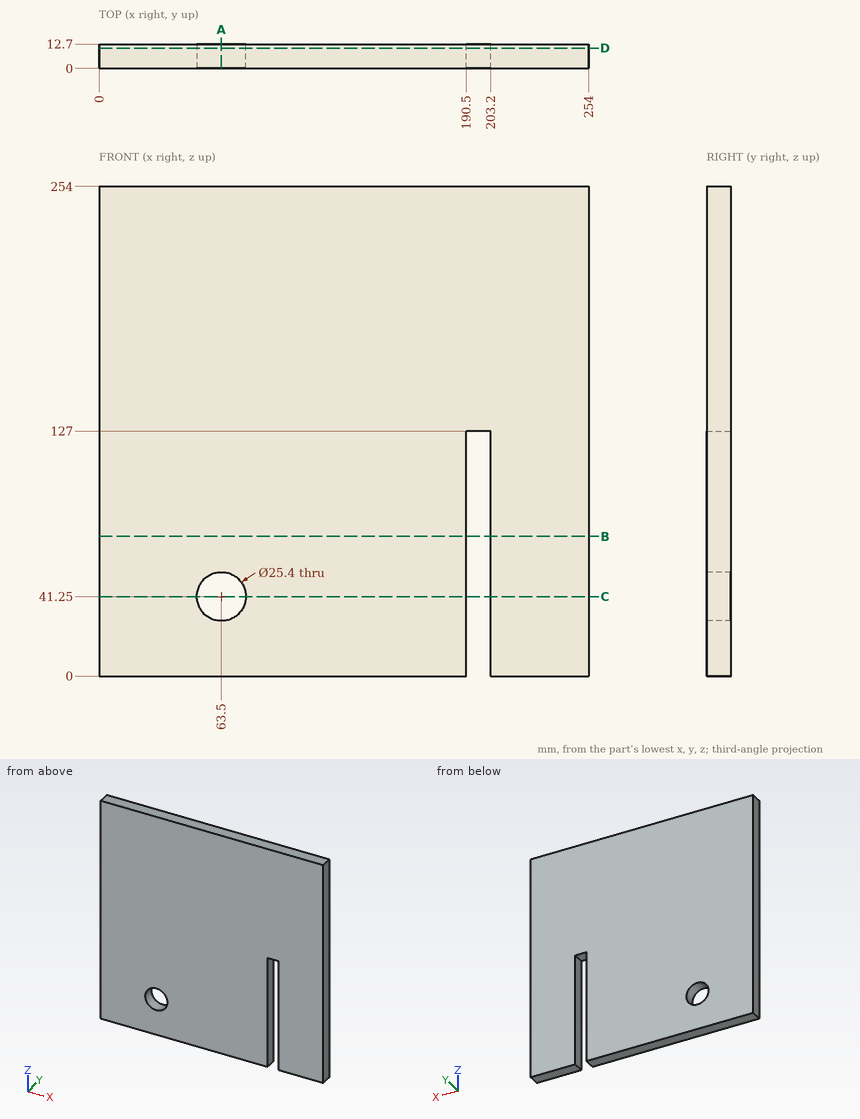
The figure shows three views and two pictorial views of one solid part (mm, origin at its lowest corner). Answer the questions. Coordinates: 2 decimals unless noted, no trailing zeros. Write each loop counter-clockwise with the first axis right and the second up, starting at its lowest first coordinate (ties: lowest second). Pieces come first, ordered by that corner, then holes. Notation, with made-up numbers: (-4, 61) -> (43, 61) arc R24 cw to (43, 71) -> close; hole circle Ø9 at (-38.75, 3). An arc over 180 degrees is marked (long way). Answer as a JSON object with one key per item and string values.
Q1. The part is cut by section A-A on x = 63.5. Give the vertices of the cut face in (y, z).
The answers:
{"outline": "(0, 0) -> (12.7, 0) -> (12.7, 28.55) -> (0, 28.55) -> close; (0, 53.95) -> (12.7, 53.95) -> (12.7, 254) -> (0, 254) -> close"}
Q2. Flat-ended cylindrical pins translate along their axes: pin 1 Ø20.5 at (x, z) = (63.5, 41.25) entering from -Y; pin 2 Ø6.5 at (x, y) = (199.5, 7) entering from -Z. Find the tip coordinate at first contact, or state that the pin passes through.
The answers:
{"pin 1": "passes through", "pin 2": "stops at z = 127"}
Q3. The part is cut by section B-B on z = 72.5. Give the vertices of the cut face in (x, y), then the cut area to 3 significant figures.
The answers:
{"outline": "(0, 0) -> (190.5, 0) -> (190.5, 12.7) -> (0, 12.7) -> close; (203.2, 0) -> (254, 0) -> (254, 12.7) -> (203.2, 12.7) -> close", "area": "3,060 mm2"}
Q4. The part is cut by section D-D on y = 10.5. Give the vertices of the cut face in (x, z), then the cut area to 3 significant figures.
The answers:
{"outline": "(0, 0) -> (190.5, 0) -> (190.5, 127) -> (203.2, 127) -> (203.2, 0) -> (254, 0) -> (254, 254) -> (0, 254) -> close; hole circle Ø25.4 at (63.5, 41.25)", "area": "62,400 mm2"}
Q5. The part is cut by section C-C on z = 41.25. Give the vertices of the cut face in (x, y), then the cut area to 3 significant figures.
The answers:
{"outline": "(0, 0) -> (50.8, 0) -> (50.8, 12.7) -> (0, 12.7) -> close; (76.2, 0) -> (190.5, 0) -> (190.5, 12.7) -> (76.2, 12.7) -> close; (203.2, 0) -> (254, 0) -> (254, 12.7) -> (203.2, 12.7) -> close", "area": "2,740 mm2"}
Q6. Consider line 1 (X direction, y = 3.5, z = 41.25); line 2 (Z direction, x = 63.5, y = 3); line 3 (X direction, y = 3.25, z = 62). Determine where each line is inside the solid, lowest interval first. Write a range as [from, to].
The answers:
{"line 1": "x = [0, 50.8], [76.2, 190.5], [203.2, 254]", "line 2": "z = [0, 28.55], [53.95, 254]", "line 3": "x = [0, 190.5], [203.2, 254]"}
